```python
from build123d import *

# Parameters (mm, degrees)
SKETCH_1_W          = 450
SKETCH_1_H          = 400
SKETCH_1_R          = 3.25
EXTRUDE_1_DEPTH     = 10
SKETCH_2_R          = 6
CUT_EXTRUDE_1_DEPTH = 6
SKETCH_3_R          = 3.75
SKETCH_3_R_2        = 4.25
CUT_EXTRUDE_2_DEPTH = 50
CUT_EXTRUDE_3_DEPTH = 50
SKETCH_5_R          = 3.25
CUT_EXTRUDE_4_DEPTH = 90


with BuildPart() as part:
    # 草图1 → 凸台-拉伸1 (new body)
    with BuildSketch(Plane.XY):
        Rectangle(SKETCH_1_W, SKETCH_1_H)
        with Locations((-115, 100)):
            Circle(SKETCH_1_R, mode=Mode.SUBTRACT)
        with Locations((115, 100)):
            Circle(SKETCH_1_R, mode=Mode.SUBTRACT)
        with Locations((115, -100)):
            Circle(SKETCH_1_R, mode=Mode.SUBTRACT)
        with Locations((-115, -100)):
            Circle(SKETCH_1_R, mode=Mode.SUBTRACT)
    extrude(amount=EXTRUDE_1_DEPTH)

    # 草图2 → 切除-拉伸1 (cut)
    with BuildSketch(Plane.XY.offset(10)):
        with Locations((-115, 100)):
            Circle(SKETCH_2_R)
        with Locations((115, 100)):
            Circle(SKETCH_2_R)
        with Locations((115, -100)):
            Circle(SKETCH_2_R)
        with Locations((-115, -100)):
            Circle(SKETCH_2_R)
    extrude(amount=-CUT_EXTRUDE_1_DEPTH, mode=Mode.SUBTRACT)

    # 草图3 → 切除-拉伸2 (cut)
    with BuildSketch(Plane.XY.offset(10)):
        with Locations((205, -180)):
            Circle(SKETCH_3_R)
        with Locations((205, -120)):
            Circle(SKETCH_3_R_2)
        with Locations((145, -180)):
            Circle(SKETCH_3_R_2)
        with Locations((145, 180)):
            Circle(SKETCH_3_R_2)
        with Locations((205, 120)):
            Circle(SKETCH_3_R_2)
        with Locations((205, 180)):
            Circle(SKETCH_3_R)
        with Locations((-205, 180)):
            Circle(SKETCH_3_R)
        with Locations((-205, 120)):
            Circle(SKETCH_3_R_2)
        with Locations((-145, 180)):
            Circle(SKETCH_3_R_2)
        with Locations((-145, -180)):
            Circle(SKETCH_3_R_2)
        with Locations((-205, -120)):
            Circle(SKETCH_3_R_2)
        with Locations((-205, -180)):
            Circle(SKETCH_3_R)
    extrude(amount=-CUT_EXTRUDE_2_DEPTH, mode=Mode.SUBTRACT)

    # 草图4 → 切除-拉伸3 (cut)
    with BuildSketch(Plane.XY.offset(10)):
        with BuildLine():
            Line((100, -12.5), (-100, -12.5))
            ThreePointArc((-100, -12.5), (-112.5, 0), (-100, 12.5))
            Line((-100, 12.5), (100, 12.5))
            ThreePointArc((100, 12.5), (112.5, 0), (100, -12.5))
        make_face()
        with BuildLine():
            Line((100, 47.5), (-100, 47.5))
            ThreePointArc((-100, 47.5), (-112.5, 60), (-100, 72.5))
            Line((-100, 72.5), (100, 72.5))
            ThreePointArc((100, 72.5), (112.5, 60), (100, 47.5))
        make_face()
        with BuildLine():
            Line((100, -47.5), (-100, -47.5))
            ThreePointArc((-100, -47.5), (-112.5, -60), (-100, -72.5))
            Line((-100, -72.5), (100, -72.5))
            ThreePointArc((100, -72.5), (112.5, -60), (100, -47.5))
        make_face()
        with BuildLine():
            Line((100, 127.5), (-100, 127.5))
            ThreePointArc((-100, 127.5), (-112.5, 140), (-100, 152.5))
            Line((-100, 152.5), (100, 152.5))
            ThreePointArc((100, 152.5), (112.5, 140), (100, 127.5))
        make_face()
        with BuildLine():
            Line((100, -127.5), (-100, -127.5))
            ThreePointArc((-100, -127.5), (-112.5, -140), (-100, -152.5))
            Line((-100, -152.5), (100, -152.5))
            ThreePointArc((100, -152.5), (112.5, -140), (100, -127.5))
        make_face()
    extrude(amount=-CUT_EXTRUDE_3_DEPTH, mode=Mode.SUBTRACT)

    # 草图5 → 切除-拉伸4 (cut)
    with BuildSketch(Plane.XY.offset(10)):
        with Locations((-15, 180)):
            Circle(SKETCH_5_R)
        with Locations((-45, 180)):
            Circle(SKETCH_5_R)
        with Locations((-75, 180)):
            Circle(SKETCH_5_R)
        with Locations((-105, 180)):
            Circle(SKETCH_5_R)
        with Locations((15, 180)):
            Circle(SKETCH_5_R)
        with Locations((45, 180)):
            Circle(SKETCH_5_R)
        with Locations((75, 180)):
            Circle(SKETCH_5_R)
        with Locations((105, 180)):
            Circle(SKETCH_5_R)
        with Locations((105, -180)):
            Circle(SKETCH_5_R)
        with Locations((75, -180)):
            Circle(SKETCH_5_R)
        with Locations((45, -180)):
            Circle(SKETCH_5_R)
        with Locations((15, -180)):
            Circle(SKETCH_5_R)
        with Locations((-105, -180)):
            Circle(SKETCH_5_R)
        with Locations((-75, -180)):
            Circle(SKETCH_5_R)
        with Locations((-45, -180)):
            Circle(SKETCH_5_R)
        with Locations((-15, -180)):
            Circle(SKETCH_5_R)
        with Locations((205, 12.5)):
            Circle(SKETCH_5_R)
        with Locations((205, 37.5)):
            Circle(SKETCH_5_R)
        with Locations((205, 62.5)):
            Circle(SKETCH_5_R)
        with Locations((205, 87.5)):
            Circle(SKETCH_5_R)
        with Locations((205, -87.5)):
            Circle(SKETCH_5_R)
        with Locations((205, -62.5)):
            Circle(SKETCH_5_R)
        with Locations((205, -37.5)):
            Circle(SKETCH_5_R)
        with Locations((205, -12.5)):
            Circle(SKETCH_5_R)
        with Locations((-205, -12.5)):
            Circle(SKETCH_5_R)
        with Locations((-205, -37.5)):
            Circle(SKETCH_5_R)
        with Locations((-205, -62.5)):
            Circle(SKETCH_5_R)
        with Locations((-205, -87.5)):
            Circle(SKETCH_5_R)
        with Locations((-205, 87.5)):
            Circle(SKETCH_5_R)
        with Locations((-205, 62.5)):
            Circle(SKETCH_5_R)
        with Locations((-205, 37.5)):
            Circle(SKETCH_5_R)
        with Locations((-205, 12.5)):
            Circle(SKETCH_5_R)
    extrude(amount=-CUT_EXTRUDE_4_DEPTH, mode=Mode.SUBTRACT)


solid = part.part
```
Geometry check sheet. Reference: the model listing, model coordinates, mm. A direction names the side the tool comes from. Coordinates: 2 decimals unless noted, no trailing zeros. Order: outer loops, then holes, each group sorted by start corner. A loop starts at its lowest first (then second) coordinate and runs counter-clockwise, first axis right, second up.
Item 1: Section check B-B (z = 8). Count the separate pieces of the cut face and the enclosed holes in it, plus the area to 3 significant figures.
Item 2: Scan lines: line 1 along Y through (x, z) = (-33, 2.5); line 2 along Y through (x, z) = (-115, 1.35); line 3 along X through (y, z) = (100, 1.45). Record each from-to range of solid material in increasing order.
Item 3: Tool access check on faces 1 (the cylindrical face through (112.497, -140.275, 5.07)), 2 (the flat face through (-112, 97, 4)), 3 (the flat face through (-225, -3, 5)). Record the directions out of +Z, -Z, +X, -X, +Y, -Y that give a thin tool (end or side, any length) a straight path to the whole face; none if there is none.
Item 4: Section check C-C (y = -54). Enter the section's corners in (x, z), plus the area to 3 significant figures.
Item 5: Mould release check, pull along Y, two halves, no side actions. Record for faces 4 (the cylindrical face through (-112.497, -59.725, 5.07)), 5 (the flat face through (-3, 200, 5)), 6 (the flat face through (-3, -200, 5)), 7 (the flat face through (-3, -42, 10)): released by +Y, released by -Y, zero draft, split by the parting line, or undercut.
Item 6: Section check A-A (y = 1.5). Enter the section's corners in (x, z), plus the area to 3 significant figures.
Item 7: Depth check by flat-ended pin: pin 1 (3.5 mm diameter, centred on x = 115, y = -102.5, fed in from +Z). Enter the tip coordinate at first touch or a pass-through.
Check sheet entries:
1. separate pieces: 1
1. enclosed holes: 53
1. area: 150,000 mm2
2. line 1: y = -200 to -152.5, -127.5 to -72.5, -47.5 to -12.5, 12.5 to 47.5, 72.5 to 127.5, 152.5 to 200
2. line 2: y = -200 to -103.25, -96.75 to 96.75, 103.25 to 200
2. line 3: x = -225 to -118.25, -111.75 to 111.75, 118.25 to 225
3. face 1: +Z, -Z
3. face 2: +Z
3. face 3: +Z, -Z, -X, +Y, -Y
4. outline: (-225, 0) - (-110.97, 0) - (-110.97, 10) - (-225, 10) - close; (110.97, 0) - (225, 0) - (225, 10) - (110.97, 10) - close
4. area: 2,280 mm2
5. face 4: undercut
5. face 5: released by +Y
5. face 6: released by -Y
5. face 7: zero draft
6. outline: (-225, 0) - (-112.41, 0) - (-112.41, 10) - (-225, 10) - close; (112.41, 0) - (225, 0) - (225, 10) - (112.41, 10) - close
6. area: 2,250 mm2
7. pin 1: stops at z = 4
